from build123d import *

# Parameters (mm, degrees)
F0_R      = 2
F0_R_2    = 6
F0_R_3    = 4
F1_DEPTH  = 4
F3_DEPTH  = 45
F4_R      = 4
F5_DEPTH  = 3.001
F6_W      = 18
F6_H      = 6.2
F6_W_2    = 40
F6_H_2    = 18
F7_DEPTH  = 4.001
F8_W      = 37
F8_H      = 4
F9_DEPTH  = 30
F10_R     = 2.5
F11_DEPTH = 4.001
F12_W     = 32
F12_H     = 45
F12_R     = 2.1
F13_DEPTH = 4
F14_R     = 1
F15_R     = 3
F16_R     = 2.99999


# Not quite as in the source:
# - a fillet or chamfer is up to 0.001 mm smaller than in the source, because OpenCascade refuses the exact size


with BuildPart() as f1:
    # F0 (on Front) → F1 (new body)
    with BuildSketch(Plane.XZ):
        Polygon((-40.5, -32), (-18.5, -32), (18.5, -32), (18.5, 0), (18.5, 31), (-18.5, 31), (-18.5, 6), (-40.5, 6), align=None)
        with BuildLine():
            ThreePointArc((-28.1833260933, 0), (-24.0098257239, 0.092032915), (-23.7739154785, -4.0758108617))
            ThreePointArc((-23.7739154785, -4.0758108617), (-29.0960224362, -12.9049296767), (-29.5751173341, -23.2029212089))
            ThreePointArc((-29.5751173341, -23.2029212089), (-31.4417329452, -27.2483725045), (-35.3144480282, -25.0456451244))
            ThreePointArc((-35.3144480282, -25.0456451244), (-34.9679215076, -11.6062828988), (-28.1833260933, 0))
        make_face(mode=Mode.SUBTRACT)
        with Locations((-9, -19)):
            Circle(F0_R, mode=Mode.SUBTRACT)
        with Locations((-15.5, 0)):
            Circle(F0_R, mode=Mode.SUBTRACT)
        with Locations((0, 7)):
            Circle(F0_R_2, mode=Mode.SUBTRACT)
        with Locations((15.5, 0)):
            Circle(F0_R, mode=Mode.SUBTRACT)
        with Locations((0, 23)):
            Circle(F0_R_3, mode=Mode.SUBTRACT)
    extrude(amount=F1_DEPTH)

    # F2 (on Top) → F3 (join)
    with BuildSketch(Plane.XY):
        Polygon((18.5, 0), (18.5, -1), (21.5, -1), (21.5, -3), (58.5, -3), (58.5, 0), align=None)
    extrude(amount=F3_DEPTH)

    # F4 (on face) → F5 (cut, through all)
    with BuildSketch(Plane.XZ.offset(3)):
        with Locations((40, 23)):
            Circle(F4_R)
    extrude(amount=-F5_DEPTH, mode=Mode.SUBTRACT)

    # F6 (on face) → F7 (cut, through all)
    with BuildSketch(Plane.XZ.offset(4)):
        with Locations((-9.5, 23.1)):
            Rectangle(F6_W, F6_H)
        with Locations((49.5, 22.9)):
            Rectangle(F6_W, F6_H)
        with Locations((38.5, 9)):
            Rectangle(F6_W_2, F6_H_2)
    extrude(amount=-F7_DEPTH, mode=Mode.SUBTRACT)

    # F8 (on face) → F9 (join)
    with BuildSketch(Plane(origin=(0, 0, 0), x_dir=(-1, 0, 0), z_dir=(0, 1, 0))):
        with Locations((0, -30)):
            Rectangle(F8_W, F8_H)
    extrude(amount=F9_DEPTH)

    # F10 (on face) → F11 (cut, through all)
    with BuildSketch(Plane.XY.offset(-28)):
        with Locations((5.5, 22)):
            Circle(F10_R)
    extrude(amount=-F11_DEPTH, mode=Mode.SUBTRACT)

    # F12 (on face) → F13 (join)
    with BuildSketch(Plane.XY.offset(31)):
        with Locations((-2.5, -22.5)):
            Rectangle(F12_W, F12_H)
        with BuildLine():
            ThreePointArc((6.6234089411, -41.9997179658), (-5.0413076784, -39.4089782063), (-14.4456133354, -32.0376430883))
            ThreePointArc((-14.4456133354, -32.0376430883), (-13.9930410249, -27.8021990866), (-9.7612789693, -28.2879948179))
            ThreePointArc((-9.7612789693, -28.2879948179), (-2.2263981239, -34.1010464578), (7.1005801395, -35.9914102312))
            ThreePointArc((7.1005801395, -35.9914102312), (10.2089825884, -39.2613770976), (6.6234089411, -41.9997179658))
        make_face(mode=Mode.SUBTRACT)
        with Locations((6.5, -15)):
            Circle(F12_R, mode=Mode.SUBTRACT)
    extrude(amount=F13_DEPTH)

    # F14
    f14_edges = [f1.edges().sort_by_distance(p)[0] for p in [
        (6, -2, 7),
        (-6, 0, 7),
        (-6, -4, 7),
        (3.996861, -4, 22.841575),
        (-2.4, -2, 26.2),
        (3.996861, 0, 22.841575),
        (-2.645751, -2, 20),
        (-10.45, -4, 26.2),
        (-18.5, -2, 26.2),
        (-10.45, 0, 26.2),
        (-10.572876, 0, 20),
    ]]
    fillet(f14_edges, radius=F14_R)

    # F15
    f15_edges = [f1.edges().sort_by_distance(p)[0] for p in [
        (0, 0, -28),
        (-40.5, -2, 6),
        (-40.5, -2, -32),
        (18.5, 30, -30),
        (-18.5, 30, -30),
        (58.5, -1.5, 45),
        (-18.5, -45, 33),
        (13.5, -45, 33),
    ]]
    fillet(f15_edges, radius=F15_R)

    # F16 (radius 3 in the source; OpenCascade refuses exactly that, so slightly less here)
    f16_edges = [f1.edges().sort_by_distance(p)[0] for p in [
        (-2.5, -4, 31),
        (-18.5, -2, 6),
    ]]
    fillet(f16_edges, radius=F16_R)


solid = f1.part
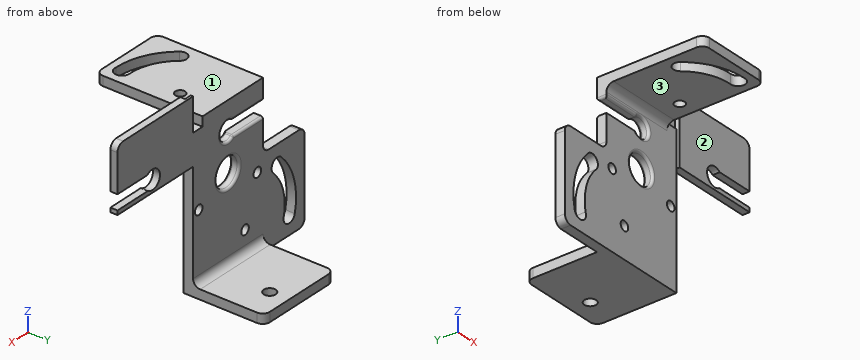
Verification items for the finished model (mm, model axes). Face numbers are marked on the shaded views. A direction names the side the tool comes from. Coordinates: 2 decimals unless noted, no trailing zeros. Write each loop counter-clockwise with the first axis right and the second up, starting at its lowest first coordinate (ties: lowest second). Pieces come first, ordered by that corner, then holes. Notation, with made-up numbers: (11.5, 58.25) - (25.5, 58.25) arc R18 cw to (25.5, 66.25) - close; hole circle Ø9 at (24.5, 74.5). An arc over 180 degrees is marked (long way). Answer as a JSON object with one key per item and string values.
(1) Cross-section at C-C on z = 23. Record the cut outline in (x, y).
Report:
{"outline": "(4, -3) arc R1 ccw to (5, -4) - (18.5, -4) - (18.5, -1) - (21.5, -1) - (21.5, -3) - (36, -3) - (36, 0) - (5, 0) arc R1 ccw to (4, -1) - close"}
(2) Cross-section at A-A on y = 22. Record the cut outline in (x, z), plus the area to 3 significant figures.
Report:
{"outline": "(-18.5, -32) - (3, -32) - (3, -28) - (-18.5, -28) - close; (8, -32) - (18.5, -32) - (18.5, -28) - (8, -28) - close", "area": "128 mm^2"}
(3) Cross-section at B-B on z = -19. Record the cut outline in (x, y), plus the area to 3 significant figures.
Report:
{"outline": "(-40.5, -4) - (-36, -4) - (-36, 0) - (-40.5, 0) - close; (-30, -4) - (-11, -4) - (-11, 0) - (-30, 0) - close; (-7, -4) - (18.5, -4) - (18.5, 0) - (-7, 0) - close", "area": "196 mm^2"}
(4) Gauge pin test, flat ends, axial feed: pin 1 Ø5.5 at (y, z) = (18, -28) entering from -X; pin 2 Ø5 at (x, z) = (-32.37, -24.37) entering from -Y; pin 3 Ø1.2 at (x, y) = (16, -1.5) entering from +Z; pin 4 Ø1 at (x, z) = (33.5, 34) entering from -Y. Record the tip position at first contact, or that the pin passes through.
Report:
{"pin 1": "x = -18.5", "pin 2": "through", "pin 3": "z = 31", "pin 4": "y = -3"}
(5) Cross-section at D-D on x = 28. Record the cut outline in (y, z), plus the area to 3 significant figures.
Report:
{"outline": "(-3, 18) - (0, 18) - (0, 45) - (-3, 45) - close", "area": "81.0 mm^2"}
(6) Thickness scan on line 1 along Y through (x, z) = (6.5, 33.2); line 2 along Z through (x, y) = (0, -2); line 3 along Z through (x, y) = (15.5, -3). Record the ranges inside material, lowest first.
Report:
{"line 1": "-45 to -42, -36 to -17.1, -12.9 to 0", "line 2": "-32 to 1, 13 to 19, 27 to 35", "line 3": "-32 to -2, 2 to 31"}
(7) Tool access check on the marked faces 1, 2 and 3. Record the directions out of +Z, -Z, +X, -X, +Y, -Y that give a thin tool (end or side, any length) a straight path to the whole face; none if there is none.
Report:
{"face 1": "+Z, -X, +Y, -Y", "face 2": "+Z, -Z, +X, -Y", "face 3": "-Z, +X, -X, -Y"}
